Input: part model. Units: mm. Frame: model coordinates. Give positions to 0.01 mm unless a question says otherwise; leave off trailing zeros. Write each loop counter-clockwise with the first axis right and the second up, starting at its lowest first coordinate (ties: lowest second). Pieces come first, ordered by that corner, then holes. Notation, with made-up numbers: (42.25, 64.5) - (80.25, 64.5) arc R12 cw to (80.25, 73.5) - close; hole circle Ø6 at (71, 23.5). An arc over 180 degrees is marked (long way). Answer as CSV lines item,"result".
```python
from build123d import *

# Parameters (mm, degrees)
SKETCH_1_R          = 4
EXTRUDE_1_DEPTH     = 175.5
SKETCH_2_R          = 2.1
CUT_EXTRUDE_1_DEPTH = 6
SKETCH_3_R          = 2.1
CUT_EXTRUDE_2_DEPTH = 6


with BuildPart() as part:
    # ｽｹｯﾁ1 → ﾎﾞｽ - 押し出し1 (new body)
    with BuildSketch(Plane(origin=(0, 0, 0), x_dir=(1, 0, 0), z_dir=(0, 1, 0))):
        Circle(SKETCH_1_R)
    extrude(amount=EXTRUDE_1_DEPTH)

    # ｽｹｯﾁ2 → ｶｯﾄ - 押し出し1 (cut)
    with BuildSketch(Plane(origin=(0, 175.5, 0), x_dir=(1, 0, 0), z_dir=(0, 1, 0))):
        Circle(SKETCH_2_R)
    extrude(amount=-CUT_EXTRUDE_1_DEPTH, mode=Mode.SUBTRACT)

    # ｽｹｯﾁ3 → ｶｯﾄ - 押し出し2 (cut)
    with BuildSketch(Plane.XZ):
        Circle(SKETCH_3_R)
    extrude(amount=-CUT_EXTRUDE_2_DEPTH, mode=Mode.SUBTRACT)


solid = part.part
```
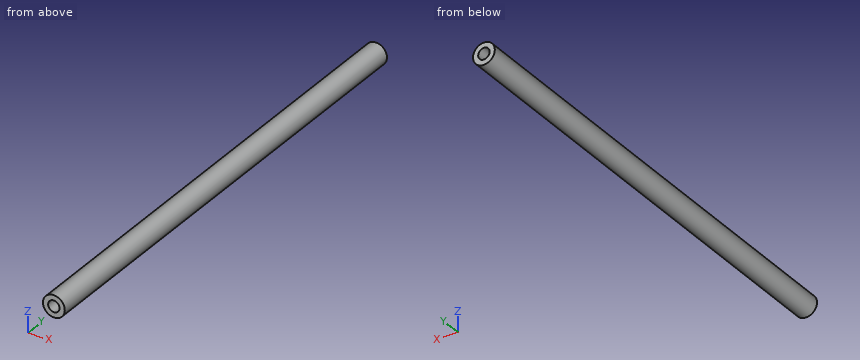
Item 1: Cut plane A-A on z = 0. Return the cut outline in (x, y), plus the area to 3 significant figures.
The answers:
outline,"(-4, 0) - (-2.1, 0) - (-2.1, 6) - (2.1, 6) - (2.1, 0) - (4, 0) - (4, 175.5) - (2.1, 175.5) - (2.1, 169.5) - (-2.1, 169.5) - (-2.1, 175.5) - (-4, 175.5) - close"
area,"1,350 mm²"
Item 2: Contact query for flat-ended pins moving along their axis: pin 1 (1.5 mm diameter, centred on x = 0.5, y = 59, fed in from +Z); pin 2 (1.5 mm diameter, centred on x = -2.5, y = 29, fed in from +Z); pin 3 (2 mm diameter, centred on x = 0.5, z = -0.5, fed in from -Y); pin 4 (3 mm diameter, centred on x = -2.5, y = 52, fed in from +Z). Output: stop coordinate, or through.
The answers:
pin 1,"z = 4"
pin 2,"z = 3.6"
pin 3,"y = 6"
pin 4,"z = 3.87"
Item 3: Ray query, line 1 (Z direction, x = 0, y = 174.1); line 2 (Z direction, x = -0.5, y = 138). Return the intervals inside material, ascending. Write a range as from..to.
The answers:
line 1,"-4..-2.1, 2.1..4"
line 2,"-3.97..3.97"
Item 4: Cut plane B-B on x = 0. Return the cut outline in (y, z), plus the area to 3 significant figures.
The answers:
outline,"(0, -4) - (175.5, -4) - (175.5, -2.1) - (169.5, -2.1) - (169.5, 2.1) - (175.5, 2.1) - (175.5, 4) - (0, 4) - (0, 2.1) - (6, 2.1) - (6, -2.1) - (0, -2.1) - close"
area,"1,350 mm²"
Item 5: Cut plane C-C on y = 151.5. Return the cut outline in (x, z).
The answers:
outline,"circle Ø8 at (0, 0)"
